Print and shaded views of the part. All mm, measured from the part's lowest x, y and z. Round coordinates to 2 decimals unless told otherwise and drop trailing zeros. Loops run counter-clockwise (first coordinate to the right, second up) from the corner with the lowest first, then second, coordinate; pieces in that order, holes last. Notation, with made-up numbers: (-27.5, 8) -> (24.5, 8) arc R5 cw to (24.5, 15) -> close; hole circle Ø5 at (1, 9.25). An arc over 180 degrees is marked (long way). Answer as CSV lines item,"result".
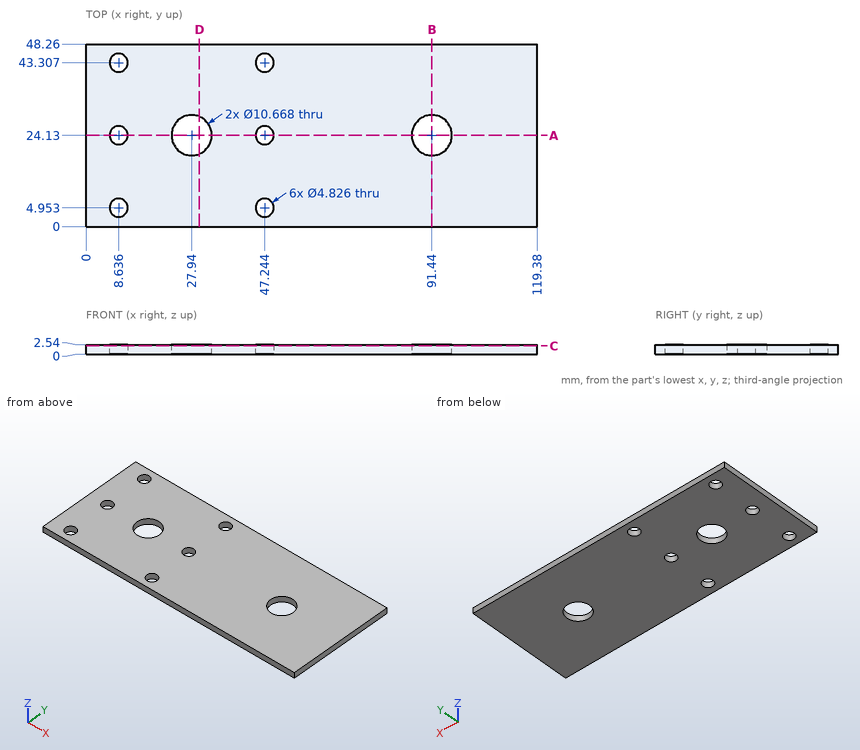
Q1. Slice it at D-D, the plane x = 30. Give the cut face in (y, z).
Results:
outline,"(0, 0) -> (19.21, 0) -> (19.21, 2.54) -> (0, 2.54) -> close; (29.05, 0) -> (48.26, 0) -> (48.26, 2.54) -> (29.05, 2.54) -> close"
Q2. Probe L1, parallel to X at y = 6.5, z = 1.3; L2, parallel to Y at x = 91.44, z = 0.85; L3, parallel to X at y = 24.5, z = 2.45. List the from-to ranges inside material, lowest first. Write a range as [from, to].
Results:
L1,"[0, 6.78], [10.49, 45.39], [49.1, 119.38]"
L2,"[0, 18.8], [29.46, 48.26]"
L3,"[0, 6.25], [11.02, 22.62], [33.26, 44.86], [49.63, 86.12], [96.76, 119.38]"
Q3. Slice it at C-C, the plane z = 2.15. Count the separate pieces of the cut face and the enclosed holes in it, and give its area (3 significant figures).
Results:
separate pieces,"1"
enclosed holes,"8"
area,"5,470 mm2"
Q4. Slice it at B-B, the plane x = 91.44. Give the cut face in (y, z).
Results:
outline,"(0, 0) -> (18.8, 0) -> (18.8, 2.54) -> (0, 2.54) -> close; (29.46, 0) -> (48.26, 0) -> (48.26, 2.54) -> (29.46, 2.54) -> close"
Q5. Slice it at A-A, the plane y = 24.13. Give the cut face in (x, z).
Results:
outline,"(0, 0) -> (6.22, 0) -> (6.22, 2.54) -> (0, 2.54) -> close; (11.05, 0) -> (22.61, 0) -> (22.61, 2.54) -> (11.05, 2.54) -> close; (33.27, 0) -> (44.83, 0) -> (44.83, 2.54) -> (33.27, 2.54) -> close; (49.66, 0) -> (86.11, 0) -> (86.11, 2.54) -> (49.66, 2.54) -> close; (96.77, 0) -> (119.38, 0) -> (119.38, 2.54) -> (96.77, 2.54) -> close"
